from build123d import *

# Parameters (mm, degrees)
SKETCH1_W              = 22.0726
SKETCH1_H              = 22.0726
BOSS_EXTRUDE1_DEPTH    = 20.32
F_10_CLEARANCE_HOLE1_D = 4.9784
SKETCH8_R              = 2.4765
CUT_EXTRUDE1_DEPTH     = 32.967201761
CUT_EXTRUDE2_DEPTH     = 6.35


with BuildPart() as part:
    # Sketch1 → Boss-Extrude1 (new body)
    with BuildSketch(Plane(origin=(0, 0, 0), x_dir=(1, 0, 0), z_dir=(0, 1, 0))):
        Rectangle(SKETCH1_W, SKETCH1_H)
    extrude(amount=BOSS_EXTRUDE1_DEPTH)

    # #10 Clearance Hole1 (through all)
    with Locations(Plane(origin=(0, 0, 0), x_dir=(-1, 0, 0), z_dir=(0, -1, 0))):
        with Locations((0, 0)):
            Hole(F_10_CLEARANCE_HOLE1_D / 2)

    # Sketch8 → Cut-Extrude1 (cut, through all)
    with BuildSketch(Plane(origin=(11.0363, 0, 0), x_dir=(0, 0, -1), z_dir=(1, 0, 0))):
        with Locations((-7.14375, 7.62)):
            Circle(SKETCH8_R)
        with Locations((7.14375, 7.62)):
            Circle(SKETCH8_R)
    extrude(amount=-CUT_EXTRUDE1_DEPTH, mode=Mode.SUBTRACT)

    # Sketch9 → Cut-Extrude2 (cut)
    with BuildSketch(Plane(origin=(0, 20.32, 0), x_dir=(1, 0, 0), z_dir=(0, 1, 0))):
        Polygon((0, 5.499261314), (-4.7625, 2.749630657), (-4.7625, -2.749630657), (0, -5.499261314), (4.7625, -2.749630657), (4.7625, 2.749630657), align=None)
    extrude(amount=-CUT_EXTRUDE2_DEPTH, mode=Mode.SUBTRACT)


solid = part.part
Model file for the job. Use its own axes, mm. A direction names the side the tool comes from. Coordinates: 2 decimals unless noted, no trailing zeros. Order: outer loops, then holes, each group sorted by start corner. A loop starts at its lowest first (then second) coordinate and runs counter-clockwise, first axis right, second up. Notation, with made-up numbers: M 3.5,23.25 L 37.5,23.25 A20 ccw 37.5,55.25 Z; hole C 27.5,8.5 d10. An arc over 180 degrees is marked long. Return JSON: item names as keys, results as strings.
1. Flat gauge pins, fed straight in: pin 1 (3 mm diameter, centred on x = -1.5, z = -2, fed in from +Y); pin 2 (8 mm diameter, centred on y = 7.62, z = -7.14, fed in from +X); pin 3 (4 mm diameter, centred on y = 7.62, z = 7.14, fed in from -X). Where does each tip first touch, or does it go through?
Ans:
{"pin 1": "y = 13.97", "pin 2": "x = 11.04", "pin 3": "through"}
2. Saw through at B-B (z = 0). Give the cut face in (x, y), and give its area (3 significant figures).
Ans:
{"outline": "M -11.04,0 L -2.49,0 L -2.49,13.97 L -4.76,13.97 L -4.76,20.32 L -11.04,20.32 Z; M 2.49,0 L 11.04,0 L 11.04,20.32 L 4.76,20.32 L 4.76,13.97 L 2.49,13.97 Z", "area": "318 mm^2"}
3. Saw through at D-D (x = -8.25). Give the cut face in (y, z), and give its area (3 significant figures).
Ans:
{"outline": "M 0,-11.04 L 20.32,-11.04 L 20.32,11.04 L 0,11.04 Z; hole C 7.62,-7.14 d4.95; hole C 7.62,7.14 d4.95", "area": "410 mm^2"}
4. Saw through at A-A (y = 7.62). Give the cut face in (x, z), and give its area (3 significant figures).
Ans:
{"outline": "M -11.04,-11.04 L 11.04,-11.04 L 11.04,-9.62 L -11.04,-9.62 Z; M -11.04,-4.67 L 11.04,-4.67 L 11.04,4.67 L -11.04,4.67 Z; M -11.04,9.62 L 11.04,9.62 L 11.04,11.04 L -11.04,11.04 Z; hole C 0,0 d4.98", "area": "249 mm^2"}
5. Tool access for faces 1 (the face through (4.762, 17, 0)), 2 (the face through (2.374, 7.083, -0.748)): list every direction of +Z, -Z, +X, -X, +Y, -Y with a clear straight run to the whole face (end or side of a thin tool).
Ans:
{"face 1": "+Y", "face 2": "+Y, -Y"}
6. Pull direction Y, two halves, no side cores. Call faces 3 (the face through (-5, 20.32, 0)), 4 (the face through (0.15, 6.11, -5.18)), 5 (the face through (-11.036, 10, 0)): +Y half, -Y half, draft (parallel to the pull), parting line (faces both ways), or undercut.
Ans:
{"face 3": "+Y half", "face 4": "undercut", "face 5": "draft"}
7. Saw through at C-C (y = 18.75). Give the cut face in (x, z).
Ans:
{"outline": "M -11.04,-11.04 L 11.04,-11.04 L 11.04,11.04 L -11.04,11.04 Z; hole M -4.76,-2.75 L 0,-5.5 L 4.76,-2.75 L 4.76,2.75 L 0,5.5 L -4.76,2.75 Z"}
8. Drill centre lines: probe 1 along Z at (x, y) = (2, 8.5); probe 2 along Z at (x, y) = (-4.5, 8.25); probe 3 along Z at (x, y) = (5.5, 8.75). Where is each one in solid material? Low to high.
Ans:
{"probe 1": "-11.04 to -9.46, -4.83 to -1.48, 1.48 to 4.83, 9.46 to 11.04", "probe 2": "-11.04 to -9.54, -4.75 to 4.75, 9.54 to 11.04", "probe 3": "-11.04 to -9.35, -4.94 to 4.94, 9.35 to 11.04"}
